Design review of the part built by this model. Coordinates are the model's own, in mm. Coordinates: 2 decimals unless noted, no trailing zeros. Write each loop counter-clockwise with the first axis right and the second up, starting at its lowest first coordinate (ties: lowest second). Pieces come first, ordered by that corner, then holes. Notation, with made-up numbers: (27.25, 88) - (44.25, 88) arc R24 cw to (44.25, 121) - close; hole circle Ø11 at (68, 56.5). An arc over 180 degrees is marked (long way). Answer as a JSON object with one key per item and string values.
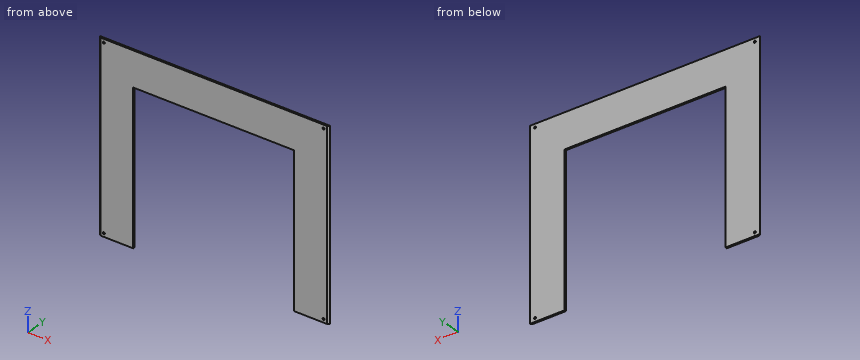
```python
from build123d import *

# Parameters (mm, degrees)
F1_DEPTH = 60
F2_DEPTH = 320
F3_R     = 1.7
F4_DEPTH = 3


with BuildPart() as f1:
    # F0 (on Top) → F1 (new body)
    with BuildSketch(Plane.XY):
        Polygon((140, 1.5), (0, 1.5), (-140, 1.5), (-140, 0), (-140, -1.5), (0, -1.5), (140, -1.5), (140, 0), align=None)
    extrude(amount=-F1_DEPTH)

    # F0 (on Top) → F2 (join)
    with BuildSketch(Plane.XY):
        Polygon((-140, 0), (-140, 1.5), (-200, 1.5), (-197, -1.5), (-140, -1.5), align=None)
        Polygon((200, 1.5), (140, 1.5), (140, 0), (140, -1.5), (197, -1.5), align=None)
    extrude(amount=-F2_DEPTH)

    # F3 (on face) → F4 (cut)
    with BuildSketch(Plane.XZ.offset(1.5)):
        with Locations((191, -6)):
            Circle(F3_R)
        with Locations((191, -314)):
            Circle(F3_R)
        with Locations((-191, -314)):
            Circle(F3_R)
        with Locations((-191, -6)):
            Circle(F3_R)
    extrude(amount=-F4_DEPTH, mode=Mode.SUBTRACT)


solid = f1.part
```
(1) Take a section at B-B, the plane y = -1.05. Write out the cut boundary in (x, z), and give its area (3 significant figures).
Solved:
{"outline": "(-197.45, -320) - (-140, -320) - (-140, -60) - (140, -60) - (140, -320) - (197.45, -320) - (197.45, 0) - (-197.45, 0) - close; hole circle Ø3.4 at (-191, -314); hole circle Ø3.4 at (-191, -6); hole circle Ø3.4 at (191, -314); hole circle Ø3.4 at (191, -6)", "area": "53,500 mm^2"}
(2) For pin 1 (3 mm diameter, centred on x = 191, z = -314, fed in from +Y); pin 2 (1.5 mm diameter, centred on x = 4.5, y = 0, fed in from +Z); pin 3 (1.5 mm diameter, centred on x = 42.5, y = 0, fed in from -Z); pin 4 (1.5 mm diameter, centred on y = -0.5, z = -181.5, fed in from -X), all flat-tipped, find the tip position at first contact; note any pin that passes through.
Solved:
{"pin 1": "passes through", "pin 2": "stops at z = 0", "pin 3": "stops at z = -60", "pin 4": "stops at x = -198.75"}
(3) Take a section at C-C, the plane x = -62. Write out the cut boundary in (y, z).
Solved:
{"outline": "(-1.5, -60) - (1.5, -60) - (1.5, 0) - (-1.5, 0) - close"}
(4) Take a section at A-A, the plane z = -191.5. Write out the cut boundary in (x, y).
Solved:
{"outline": "(-200, 1.5) - (-197, -1.5) - (-140, -1.5) - (-140, 1.5) - close; (140, -1.5) - (197, -1.5) - (200, 1.5) - (140, 1.5) - close"}
(5) To check wall thickness, follow line 1 (Z direction, x = 191, y = -0.3); line 2 (Z direction, x = -71, y = 0.75); line 3 (X direction, y = -0.1, z = -231.5). State the ranges of each line that lie inside material, in increasing order. Write a range as from..to.
Solved:
{"line 1": "z = -320..-315.7, -312.3..-7.7, -4.3..0", "line 2": "z = -60..0", "line 3": "x = -198.4..-140, 140..198.4"}
